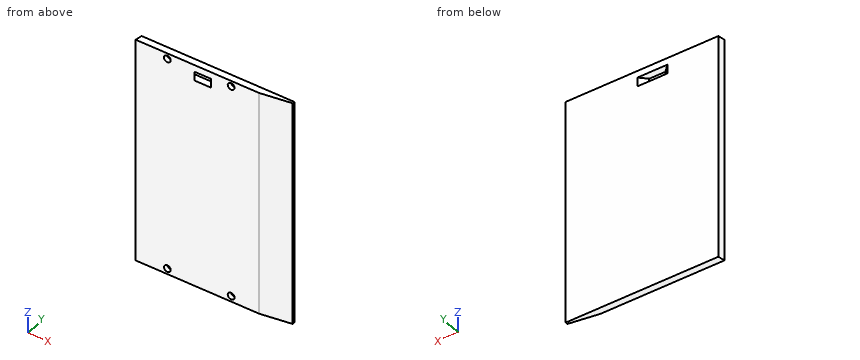
Autodesk Inventor part; units mm, degrees
ref_plane "YZ Plane" through (0, 0, 0) normal (1, 0, 0) x (0, 1, 0)
ref_plane "XZ Plane" through (0, 0, 0) normal (0, 1, 0) x (-1, 0, 0)
ref_plane "XY Plane" through (0, 0, 0) normal (0, 0, 1) x (1, 0, 0)
sketch "Sketch1" plane through (0, 0, 0) normal (0, 0, 1) x (1, 0, 0)
  line L0 (-24.865, 1.7403) -> (-25.3518, -1.2597)
  line L1 (-25.3518, -1.2597) -> (28.8493, -1.2597)
  line L2 (-24.865, 1.7403) -> (42.135, 1.7403)
  line L3 (42.135, 1.7403) -> (42.135, 0.7403)
  line L4 (42.135, 0.7403) -> (28.8493, -1.2597)
  point P0 (0, 0)
  dimension "d0" = 67
  dimension "d26" = 3
  dimension "d27" = 1
  dimension "d46" = 0.4868
  dimension "d48" = 13.2857
extrude "Extrusion1" add sketch "Sketch1" along normal blind 100
sketch "Sketch3" plane through (-24.865, 1.7403, 0) normal (0, 1, 0) x (1, 0, 0)
  line L0 (25.3402, -93) -> (32.491, -93)
  line L1 (32.491, -93) -> (32.491, -97)
  line L2 (32.491, -97) -> (25.3402, -97)
  line L3 (25.3402, -97) -> (25.3402, -93)
  line L4 (-0.4868, 0) -> (-0.4868, -100)
  point P0 (24.865, 0)
  point P1 (16.7856, -97)
  point P2 (23.8348, -93)
  dimension "d49" = 25.827
  dimension "d50" = 7.1508
extrude "Extrusion2" cut sketch "Sketch3" against normal through all
chamfer "Chamfer2" distance 3 angle 45 2 edges at (0.4752, 1.7403, 95) (7.626, 1.7403, 95) measured on face at (8.2987, 1.7403, 31)
sketch "Sketch4" plane through (-25.3518, -1.2597, 0) normal (0, -1, 0) x (1, 0, 0)
  circle A0 centre (13.887, 97.5) radius 1.5
  circle A1 centre (41.887, 97.5) radius 1.5
  circle A2 centre (13.887, 2.5) radius 1.5
  circle A3 centre (41.887, 2.5) radius 1.5
  line L0 (0, 100) -> (54.2011, 100)
  line L1 (0, 0) -> (54.2011, 0)
  line L2 (0, 0) -> (0, 100)
  point P0 (25.3518, 0)
  dimension "d28" = 3
  dimension "d29" = 3
  dimension "d30" = 3
  dimension "d31" = 3
  dimension "d32" = 2.5
  dimension "d33" = 2.5
  dimension "d34" = 2.5
  dimension "d35" = 2.5
  dimension "d36" = 13.887
  dimension "d37" = 28
  dimension "d38" = 13.887
  dimension "d39" = 28
extrude "Extrusion3" cut sketch "Sketch4" against normal blind 2
properties part number "porywa" material "Polycarbonate, Clear"
Can you work these out from the model? Positions are in its coordinate system, mm. Give positions to 0.01 mm unless a question says otherwise; leave off trailing zeros. Write each loop counter-clockwise with the first axis right and the second up, starting at its lowest first coordinate (ties: lowest second). Pieces come first, ordered by that corner, then holes. Notation, with made-up numbers: (-12.5, -13.5) -> (32.5, -13.5) arc R19 ccw to (32.5, 0.5) -> close; hole circle Ø4 at (9, -18). An arc over 180 degrees is marked (long way). Answer as a JSON object with one key per item and string values. Group by question number.
Item 1: Please list where these lines run through material, in increasing order: line 1 (Z direction, x = 6, y = 1.6); line 2 (Y direction, x = 29, z = 31); line 3 (X direction, y = 0.85, z = 66) (3 decimals). Write a range as [from, to].
Item 2: Suppose I cut it at C-C (z = 2.5). Please give me the cut outline in (x, y) (3 decimals).
Item 3: Suppose I cut it at B-B (y = -0.5). Please give me the cut outline in (x, z), plus the area to 3 significant figures.
Item 4: Suppose I cut it at A-A (z = 90.5). Please give me the cut outline in (x, y) (3 decimals).
Item 5: I'm going to push a flat-ended pin straight in: P1, Ø2.5, axis at x = -12, z = 2.5, coming from the -Y side. Where does the tip first touch, or does it pass through?
Findings:
{
 "1": {"line 1": "z = [0, 93], [97, 100]", "line 2": "y = [-1.24, 1.74]", "line 3": "x = [-25.009, 42.135]"},
 "2": {"outline": "(-25.352, -1.26) -> (-12.965, -1.26) -> (-12.965, 0.74) -> (-9.965, 0.74) -> (-9.965, -1.26) -> (15.035, -1.26) -> (15.035, 0.74) -> (18.035, 0.74) -> (18.035, -1.26) -> (28.849, -1.26) -> (42.135, 0.74) -> (42.135, 1.74) -> (-24.865, 1.74) -> close"},
 "3": {"outline": "(-25.23, 0) -> (33.9, 0) -> (33.9, 100) -> (-25.23, 100) -> close; hole circle Ø3 at (-11.46, 2.5); hole circle Ø3 at (-11.46, 97.5); hole (-0.28, 93) -> (8.39, 93) -> (8.39, 97) -> (-0.28, 97) -> close; hole circle Ø3 at (16.54, 2.5); hole circle Ø3 at (16.54, 97.5)", "area": "5,850 mm²"},
 "4": {"outline": "(-25.352, -1.26) -> (28.849, -1.26) -> (42.135, 0.74) -> (42.135, 1.74) -> (-24.865, 1.74) -> close"},
 "5": {"P1": "stops at y = -1.26"}
}
